Work out the finished part from the listing and answer in its coordinate system (mm). Coordinates: 2 decimals unless noted, no trailing zeros. Loops run counter-clockwise (first coordinate to the right, second up) from the corner with the lowest first, then second, coordinate; pieces in that order, holes last. Notation, with made-up numbers: (21.25, 55) -> (32.25, 55) arc R21 cw to (32.25, 62) -> close; hole circle Ø3 at (16, 65.25). An arc over 180 degrees is marked (long way). Answer as CSV lines item,"result".
```python
from build123d import *

# Parameters (mm, degrees)
SKETCH1_R           = 2.5
BOSS_EXTRUDE1_DEPTH = 3.18
CUT_EXTRUDE1_DEPTH  = 155.06204075


with BuildPart() as part:
    # Sketch1 → Boss-Extrude1 (new body)
    with BuildSketch(Plane(origin=(0, 0, 0), x_dir=(1, 0, 0), z_dir=(0, 1, 0))):
        Polygon((0, 0), (40, 0), (90, 0), (90, 40), (90, 85), (90, 125), (-50, 125), (-50, 0), align=None)
        with Locations(Location((-35, 115, 0), (0, 0, 90))):
            Circle(SKETCH1_R, mode=Mode.SUBTRACT)
        with Locations(Location((75, 115, 0), (0, 0, 90))):
            Circle(SKETCH1_R, mode=Mode.SUBTRACT)
        with Locations(Location((20, 95, 0), (0, 0, 90))):
            Circle(SKETCH1_R, mode=Mode.SUBTRACT)
        with Locations(Location((10, 20, 0), (0, 0, 90))):
            Circle(SKETCH1_R, mode=Mode.SUBTRACT)
        with Locations(Location((30, 20, 0), (0, 0, 90))):
            Circle(SKETCH1_R, mode=Mode.SUBTRACT)
    extrude(amount=BOSS_EXTRUDE1_DEPTH)

    # Sketch3 → Cut-Extrude1 (cut, through all)
    with BuildSketch(Plane.XZ):
        Polygon((90, -40), (50, 0), (90, 0), align=None)
        Polygon((-50, 0), (-10, 0), (-50, -40), align=None)
    extrude(amount=-CUT_EXTRUDE1_DEPTH, mode=Mode.SUBTRACT)


solid = part.part
```
(1) For a pull along Z with two mould halves and no side action, classify faces 1 (the face through (21, 2, -125)), 2 (the face through (19, 3.18, -63)), 3 (the face through (-35.751, 1.568, -117.385)), 4 (the face through (-30, 2, -20)) as pulls with the +Z half, pulls with the -Z half, needs draft (parallel to the pull), parting line crosses it, or undercut.
Computed values:
face 1,"pulls with the -Z half"
face 2,"needs draft"
face 3,"undercut"
face 4,"pulls with the +Z half"
(2) A cutting plane is placed at A-A, the plane z = -115. Write down the section's boundary in (x, y).
Computed values:
outline,"(-50, 0) -> (-37.5, 0) -> (-37.5, 3.18) -> (-50, 3.18) -> close; (-32.5, 0) -> (72.5, 0) -> (72.5, 3.18) -> (-32.5, 3.18) -> close; (77.5, 0) -> (90, 0) -> (90, 3.18) -> (77.5, 3.18) -> close"
(3) A cutting plane is placed at B-B, the plane x = 75. Write down the section's boundary in (y, z), and give its area (3 significant figures).
Computed values:
outline,"(0, -125) -> (3.18, -125) -> (3.18, -117.5) -> (0, -117.5) -> close; (0, -112.5) -> (3.18, -112.5) -> (3.18, -25) -> (0, -25) -> close"
area,"302 mm2"
(4) A cutting plane is placed at C-C, the plane y = 1. Write down the section's boundary in (x, z).
Computed values:
outline,"(-50, -125) -> (90, -125) -> (90, -40) -> (50, 0) -> (-10, 0) -> (-50, -40) -> close; hole circle Ø5 at (-35, -115); hole circle Ø5 at (10, -20); hole circle Ø5 at (20, -95); hole circle Ø5 at (30, -20); hole circle Ø5 at (75, -115)"
(5) Consider line 1 along X through (y, z) = (1.55, -115); line 2 along Z through (x, y) = (30, 1.5); line 3 along X through (y, z) = (1.8, -20). Determine where each line is inside the solid, lowest interval first.
Computed values:
line 1,"-50 to -37.5, -32.5 to 72.5, 77.5 to 90"
line 2,"-125 to -22.5, -17.5 to 0"
line 3,"-30 to 7.5, 12.5 to 27.5, 32.5 to 70"
(6) A cutting plane is placed at D-D, the plane x = 30. Write down the section's boundary in (y, z), and give its area (3 significant figures).
Computed values:
outline,"(0, -125) -> (3.18, -125) -> (3.18, -22.5) -> (0, -22.5) -> close; (0, -17.5) -> (3.18, -17.5) -> (3.18, 0) -> (0, 0) -> close"
area,"382 mm2"
(7) Flat-ended cylindrical pins translate along their axes: pin 1 Ø6.5 at (x, z) = (-35, -115) entering from +Y; pin 2 Ø1 at (y, z) = (2, -16) entering from +X. Find the tip coordinate at first contact, or state that the pin passes through.
Computed values:
pin 1,"y = 3.18"
pin 2,"x = 66.5"
